Geometry: see drawing. Coordinates: mm, zero at the bounding-box minimum. Give positions to 0.01 mm unless a question says otherwise; leave off trailing zeros. Loops run counter-clockwise (first coordinate to the right, second up) from the corner with the lowest first, then second, coordinate; pieces in that order, holes last. Notation, with made-up numbers: M 74,83.5 L 126,83.5 A26 cw 126,106.5 Z; hole C 35,62 d7. An arc over 180 degrees is marked long. Put each result on its own line as item: value.
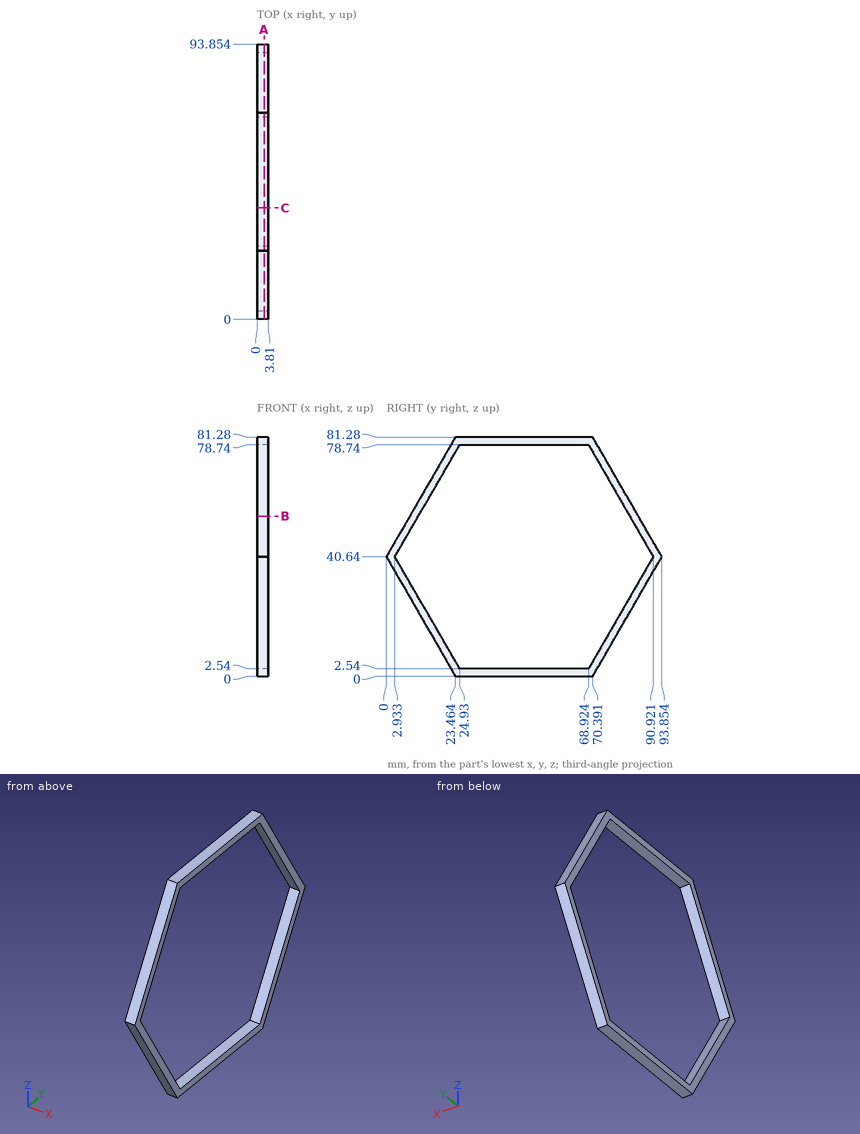
Item 1: Line query: probe 1 along Z at (x, y) = (1.85, 63); probe 2 along Y at (x, z) = (3.4, 46.5) (1 decimal); probe 3 along Y at (x, z) = (2.95, 75) (1 decimal). Output: solid intervals per line, ascending. Write a range as [from, to].
Output values:
probe 1: [0, 2.54], [78.74, 81.28]
probe 2: [3.4, 6.3], [87.5, 90.5]
probe 3: [19.8, 22.8], [71.1, 74]
Item 2: Section B-B on z = 54.5. Output: boundary loops of the cut face in (x, y) (1 decimal).
Output values:
outline: M 0,8 L 3.8,8 L 3.8,10.9 L 0,10.9 Z; M 0,82.9 L 3.8,82.9 L 3.8,85.9 L 0,85.9 Z
Item 3: Section A-A on x = 2.35. Output: boundary loops of the cut face in (y, z) (1 decimal).
Output values:
outline: M 0,40.6 L 23.5,0 L 70.4,0 L 93.9,40.6 L 70.4,81.3 L 23.5,81.3 Z; hole M 2.9,40.6 L 24.9,2.5 L 68.9,2.5 L 90.9,40.6 L 68.9,78.7 L 24.9,78.7 Z
Item 4: Section C-C on y = 38. Output: boundary loops of the cut face in (x, z).
Output values:
outline: M 0,0 L 3.81,0 L 3.81,2.54 L 0,2.54 Z; M 0,78.74 L 3.81,78.74 L 3.81,81.28 L 0,81.28 Z
